CAD build for the part. Positions are in the model's coordinates, mm. Face numbers are marked on the shaded views. Coordinates: 2 decimals unless noted, no trailing zeros. Loops run counter-clockwise (first coordinate to the right, second up) from the corner with the lowest first, then second, coordinate; pieces in that order, holes last. Notation, with made-up numbers: (59, -27.75) -> (88, -27.75) arc R34 cw to (88, 6.25) -> close; hole circle Ø1 at (33.5, 60). An arc over 180 degrees is marked (long way). Return JSON: item names as keys, results as strings. Group by question number.
(1) Flat gauge pins, fed straight in: pin 1 Ø8 at (y, z) = (-12, 19) entering from -X; pin 2 Ø2 at (x, y) = (16.5, -12) entering from -Z; pin 3 Ø4 at (y, z) = (-10.5, 16) entering from -X. Where does each tip first touch, or does it go through?
(2) Mould opens along X. For the marked faces 1, 2 and 3 say: pulls with the +X half, pulls with the -X half, needs draft (parallel to the pull), parting line crosses it, or undercut.
(3) Probe L1, parallel to Y at x = 0, z = 24.7; L2, parallel to X at y = -4.25, z = 6.25; L3, parallel to X at y = -1, z = 12.25. List the from-to ranges inside material, lowest first.
(4) Saw through at D-D on z = 4. Write the cut outline in (x, y).
(5) Saw through at A-A on x = 0. Write the cut outline in (y, z).
(6) Saw through at C-C on z = 20. Write the cut outline in (x, y).
(7) Saw through at B-B on y = -10. Write the cut outline in (x, z), then the cut area to 3 significant figures.
```python
from build123d import *

# Parameters (mm, degrees)
F1_DEPTH = 20
F2_W     = 0.5
F2_H     = 2
F4_R     = 0.9
F5_DEPTH = 25.001


with BuildPart() as f1:
    # F0 (on Front) → F1 (new body)
    with BuildSketch(Plane.XZ):
        with BuildLine():
            Line((24, 0), (25, 0))
            ThreePointArc((25, 0), (0, 25), (-25, 0))
            Line((-25, 0), (-24, 0))
            ThreePointArc((-24, 0), (0, 24), (24, 0))
        make_face()
    extrude(amount=F1_DEPTH)

    # F2 (on face) → F3 (revolve, cut)
    with BuildSketch(Plane(origin=(0, 0, 0), x_dir=(1, 0, 0), z_dir=(0, 0, -1))):
        with Locations((-24.25, 10)):
            Rectangle(F2_W, F2_H)
    revolve(axis=Axis((0, -6.667699, 0), (0, -1, 0)), mode=Mode.SUBTRACT)

    # F4 (on face) → F5 (cut, through all)
    with BuildSketch(Plane(origin=(0, 0, 0), x_dir=(1, 0, 0), z_dir=(0, 0, -1))):
        with Locations((0, 10)):
            Circle(F4_R)
    extrude(amount=-F5_DEPTH, mode=Mode.SUBTRACT)


solid = f1.part
```
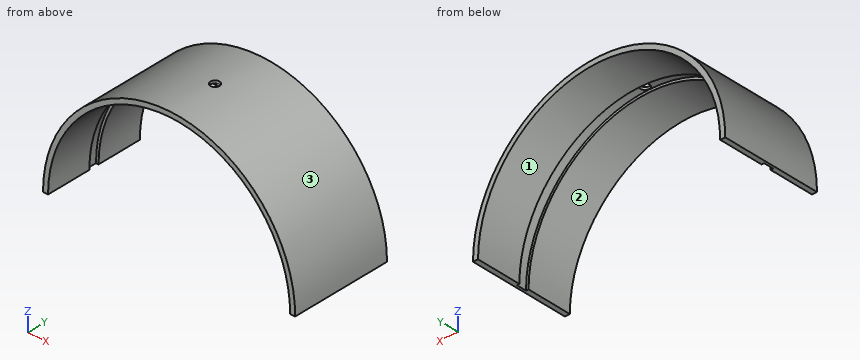
Geometry results:
{
 "1": {"pin 1": "x = -20", "pin 2": "z = 16.42", "pin 3": "x = -20.71"},
 "2": {"face 1": "undercut", "face 2": "undercut", "face 3": "parting line crosses it"},
 "3": {"L1": "-20 to -10.9, -9.1 to 0", "L2": "-24.21 to -23.17, 23.17 to 24.21", "L3": "-21.79 to -20.64, 20.64 to 21.79"},
 "4": {"outline": "(-24.68, -20) -> (-23.66, -20) -> (-23.66, -11) -> (-24.17, -11) -> (-24.17, -9) -> (-23.66, -9) -> (-23.66, 0) -> (-24.68, 0) -> close; (23.66, -20) -> (24.68, -20) -> (24.68, 0) -> (23.66, 0) -> (23.66, -9) -> (24.17, -9) -> (24.17, -11) -> (23.66, -11) -> close"},
 "5": {"outline": "(-20, 24) -> (-11, 24) -> (-11, 24.5) -> (-10.9, 24.5) -> (-10.9, 25) -> (-20, 25) -> close; (-9.1, 24.5) -> (-9, 24.5) -> (-9, 24) -> (0, 24) -> (0, 25) -> (-9.1, 25) -> close"},
 "6": {"outline": "(-15, -20) -> (-13.27, -20) -> (-13.27, -11) -> (-14.15, -11) -> (-14.15, -9) -> (-13.27, -9) -> (-13.27, 0) -> (-15, 0) -> close; (13.27, -20) -> (15, -20) -> (15, 0) -> (13.27, 0) -> (13.27, -9) -> (14.15, -9) -> (14.15, -11) -> (13.27, -11) -> close"},
 "7": {"outline": "(-25, 0) -> (-24.5, 0) arc R24.5 cw to (-0.9, 24.48) -> (-0.9, 24.98) arc R25 ccw to start; (0.9, 24.48) arc R24.5 cw to (24.5, 0) -> (25, 0) arc R25 ccw to (0.9, 24.98) -> close", "area": "38.0 mm²"}
}
